The listing builds one solid part. Answer for the finished solid, in the listing's coordinates (mm). Face numbers are marked on the shaded views. A direction names the side the tool comes from. Give positions to 0.01 mm unless a question says otherwise; leave off trailing zeros. Order: outer loops, then holes, each group sorted by start corner. A loop starts at its lowest first (then second) coordinate and runs counter-clockwise, first axis right, second up. Notation, with made-up numbers: (85.5, -30.75) - (90.5, -30.75) arc R16 ccw to (90.5, -21.75) - close; hole circle Ø5 at (-39.75, 54). An arc over 180 degrees is marked (long way). Answer in a Markdown table with one row per item.
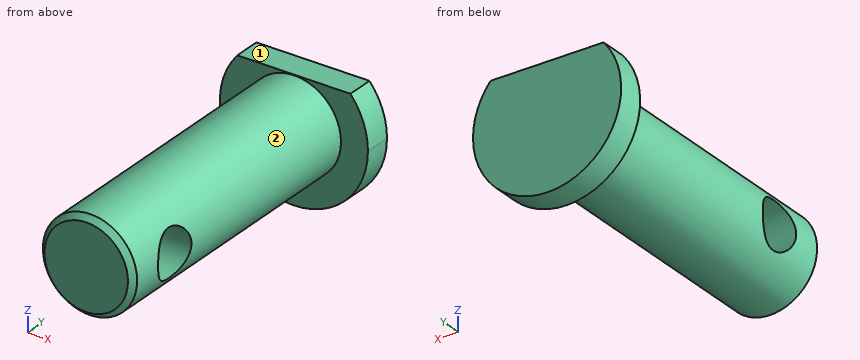
from build123d import *

# Parameters (mm, degrees)
F0_R          = 7
F1_DEPTH      = 4
F2_DEPTH      = 47.6
F3_SIZE       = 0.8
F4_R          = 3.5
F5_DEPTH      = 14.3
F5_DEPTH_BACK = 14.4


with BuildPart() as f1:
    # F0 (on Front) → F1 (new body)
    with BuildSketch(Plane.XZ):
        with BuildLine():
            ThreePointArc((-8.401786, 7.1), (-3.780235, -10.330045), (11, 0))
            ThreePointArc((11, 0), (10.330045, 3.780235), (8.401786, 7.1))
            Line((8.401786, 7.1), (-8.401786, 7.1))
        make_face()
        Circle(F0_R, mode=Mode.SUBTRACT)
    extrude(amount=F1_DEPTH)

    # F0 (on Front) → F2 (join)
    with BuildSketch(Plane.XZ):
        Circle(F0_R)
    extrude(amount=F2_DEPTH)

    # F3
    f3_edges = [f1.edges().sort_by_distance(p)[0] for p in [
        (-7, -47.6, 0),
    ]]
    chamfer(f3_edges, length=F3_SIZE)

    # F4 (on Right) → F5 (cut, two sides)
    with BuildSketch(Plane.YZ) as f5_sk:
        with Locations((-38.9, 0)):
            Circle(F4_R)
    extrude(amount=F5_DEPTH, mode=Mode.SUBTRACT)
    extrude(f5_sk.sketch, amount=-F5_DEPTH_BACK, mode=Mode.SUBTRACT)


solid = f1.part
Item 1: Find section C-C on y = -20. Write down the section's boundary in (x, z).
Answer block:
| item | result |
|---|---|
| outline | circle Ø14 at (0, 0) |
Item 2: Each of these flat-tipped pins is pushed along its axis until it touches: P1, Ø5, axis at y = -43, z = -7.5, coming from the -X side; P2, Ø2, axis at x = 4, z = -7, coming from the -Y side; P3, Ø12, axis at x = 6.5, y = -36, coming from the -Z side; P4, Ø4, axis at y = -38.9, z = 0, coming from the +X side. Where does it stop, or does it pass through?
Answer block:
| item | result |
|---|---|
| P1 | x = -4.9 |
| P2 | y = -4 |
| P3 | z = -6.98 |
| P4 | through |
Item 3: Find section B-B on z = -9.25. Write down the section's boundary in (x, y).
Answer block:
| item | result |
|---|---|
| outline | (-5.95, -4) - (5.95, -4) - (5.95, 0) - (-5.95, 0) - close |
Item 4: Find section A-A on y = -41.5. Write down the section's boundary in (x, z), then the cut area to 3 significant figures.
Answer block:
| item | result |
|---|---|
| outline | (-6.6, -2.34) arc R7 ccw to (6.6, -2.34) - close; (-6.6, 2.34) - (6.6, 2.34) arc R7 ccw to start |
| area | 89.6 mm² |
Item 5: Consider line 1 (Y direction, x = -4, z = 0); line 2 (X direction, y = -26.5, z = 3.25); line 3 (Y direction, x = -3.5, z = 3). Determine where each line is inside the solid, lowest interval first.
Answer block:
| item | result |
|---|---|
| line 1 | -47.6 to -42.4, -35.4 to 0 |
| line 2 | -6.2 to 6.2 |
| line 3 | -47.6 to -40.7, -37.1 to 0 |
Item 6: Which of the six approach directions +Z, -Z, +X, -X, +Y, -Y give full straight-line access (tool end or side, diameter ignored) to the marked faces 1 and 2?
Answer block:
| item | result |
|---|---|
| face 1 | +Z, +X, -X, +Y, -Y |
| face 2 | -Y |
